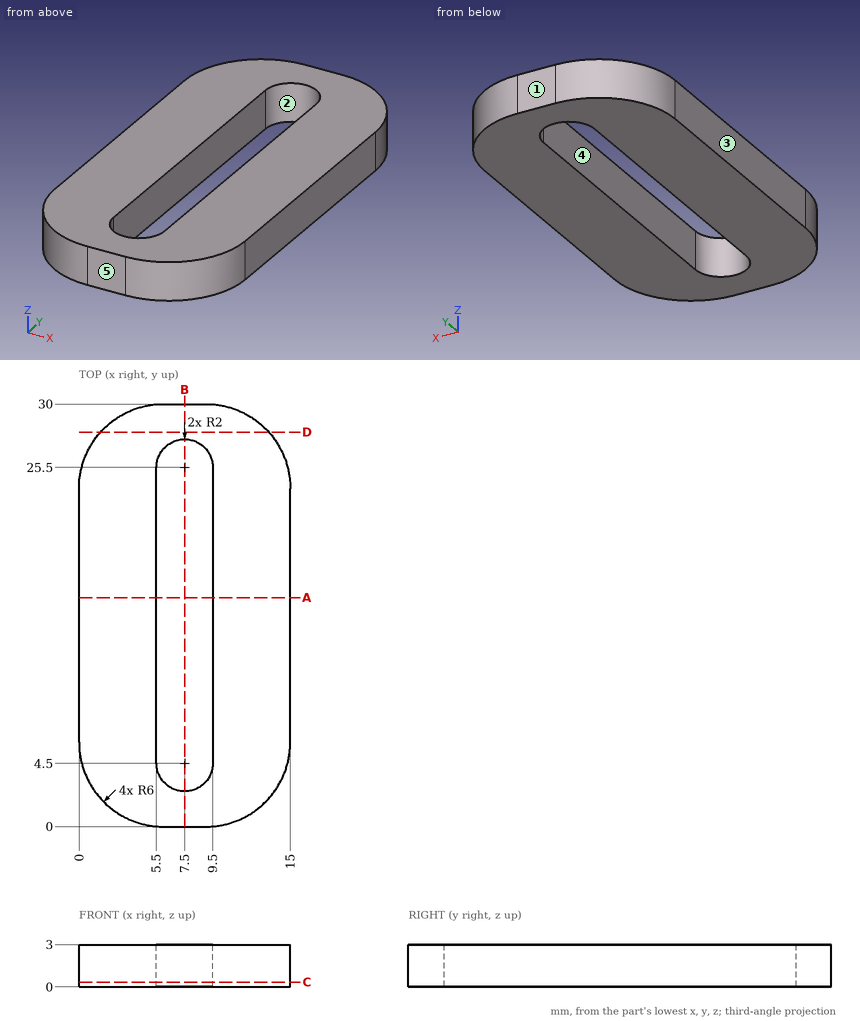
Verification items for this drawing (mm, ordinates from the low corner). A direction names the side the tool comes from. Give positions to 0.01 mm unless a question says otherwise; leave off trailing zeros. Order: outer loops, then holes, each group sorted by start corner. A loop starts at its lowest first (then second) coordinate and runs counter-clockwise, first axis right, second up. Notation, with made-up numbers: M 21.5,57 L 26.5,57 A35 ccw 26.5,92 Z; hole C 74,47.5 d1. An arc over 180 degrees is marked long. Use a Markdown table: item, result.
Item 1: Draft check along X on the marked faces 3, 4 and 5. Enter one of: +X half, -X half, draft (parallel to the pull), parting line (faces both ways), or undercut.
Answers follow:
| item | result |
|---|---|
| face 3 | -X half |
| face 4 | undercut |
| face 5 | draft |
Item 2: Section check A-A (y = 16.25). Record the cut outline in (x, z).
Answers follow:
| item | result |
|---|---|
| outline | M 0,0 L 5.5,0 L 5.5,3 L 0,3 Z; M 9.5,0 L 15,0 L 15,3 L 9.5,3 Z |
Item 3: Depth check by flat-ended pin: P1, Ø1.5, axis at x = 10.5, z = 1, coming from the -Y side; P2, Ø1.5, axis at y = 11, z = 1.5, coming from the -X side. Enter the tip coordinate at first touch or a pass-through.
Answers follow:
| item | result |
|---|---|
| P1 | stops at y = 0.05 |
| P2 | stops at x = 0 |
Item 4: Tool access check on the marked faces 1 and 2. Record the directions out of +Z, -Z, +X, -X, +Y, -Y that give a thin tool (end or side, any length) a straight path to the whole face; none if there is none.
Answers follow:
| item | result |
|---|---|
| face 1 | +Z, -Z, +X, -X, +Y |
| face 2 | +Z, -Z |
Item 5: Material ranges on line 1 along X through (y, z) = (19, 2.8); line 2 along X through (y, z) = (26.75, 1.9); line 3 along Y through (x, z) = (9, 0.35), recorded low to high.
Answers follow:
| item | result |
|---|---|
| line 1 | x = 0 to 5.5, 9.5 to 15 |
| line 2 | x = 0.67 to 5.94, 9.06 to 14.33 |
| line 3 | y = 0 to 3.18, 26.82 to 30 |
Item 6: Section check B-B (x = 7.5). Record the cut outline in (y, z).
Answers follow:
| item | result |
|---|---|
| outline | M 0,0 L 2.5,0 L 2.5,3 L 0,3 Z; M 27.5,0 L 30,0 L 30,3 L 27.5,3 Z |
Item 7: Section check C-C (z = 0.35). Record the cut outline in (x, y).
Answers follow:
| item | result |
|---|---|
| outline | M 0,6 A6 ccw 6,0 L 9,0 A6 ccw 15,6 L 15,24 A6 ccw 9,30 L 6,30 A6 ccw 0,24 Z; hole M 5.5,4.5 A2 ccw 9.5,4.5 L 9.5,25.5 A2 ccw 5.5,25.5 Z |
Item 8: Section check D-D (y = 28). Record the cut outline in (x, z), and give its area (3 significant figures).
Answers follow:
| item | result |
|---|---|
| outline | M 1.53,0 L 13.47,0 L 13.47,3 L 1.53,3 Z |
| area | 35.8 mm2 |
